Part model, mm, in its own coordinate system. Face numbers are marked on the shaded views. A direction names the side the tool comes from. Round coordinates to 2 decimals unless told otherwise and drop trailing zeros. Loops run counter-clockwise (first coordinate to the right, second up) from the corner with the lowest first, then second, coordinate; pieces in that order, holes last.
(1) Probe probe 1 along Z at (x, y) = (-0.9, 1.25); probe 2 along Z at (x, y) = (-0.65, -0.5) (3 decimals); probe 3 along Y at (x, z) = (0.4, 1.75). List the from-to ranges inside material, lowest first.
(2) Tool access for the marked faces 1 and 2: list every direction of +Z, -Z, +X, -X, +Y, -Y with a clear straight run to the whole face (end or side of a thin tool).
(3) Cut at A-A on z = -2. List the corners of the cut face in (x, y), then the cut area to 3 significant figures.
(4) Mould opens along X. For the marked faces 3, 4, 5 and 6 say: +X half, -X half, draft (parallel to the pull), parting line (faces both ways), or undercut.
(5) Flat gauge pins, fed straight in: pin 1 (1.2 mm diameter, centred on x = 0, y = 0, fed in from +Z); pin 2 (1.5 mm diameter, centred on x = -1, z = -0.5, fed in from -Y). Where does each tip first touch, or does it go through?
Autodesk Inventor part; units mm, degrees
ref_plane "YZ Plane" through (0, 0, 0) normal (1, 0, 0) x (0, 1, 0)
ref_plane "XZ Plane" through (0, 0, 0) normal (0, 1, 0) x (-1, 0, 0)
ref_plane "XY Plane" through (0, 0, 0) normal (0, 0, 1) x (1, 0, 0)
sketch "Sketch1" plane through (0, 0, 0) normal (0, 0, 1) x (1, 0, 0)
  circle A0 centre (0, 0) radius 2.3241
  dimension "max_head_dia" = 4.6482
extrude "Extrusion1" add sketch "Sketch1" along normal blind 2.8448
sketch "Sketch2" plane through (0, 0, 0) normal (0, 0, -1) x (-1, 0, 0)
  circle A0 centre (0, 0) radius 2.3241
  circle A1 centre (0, 0) radius 1.4224
  dimension "max_body_dia" = 2.8448
extrude "Extrusion2" add sketch "Sketch2" along normal blind 9.525 contours A1
sketch "Sketch3" plane through (0, 0, 2.8448) normal (0, 0, 1) x (1, 0, 0)
  circle A0 centre (0, 0) radius 2.3241
  line L0 (-1.1397, 0.7689) -> (0.096, 1.3715)
  line L1 (0.096, 1.3715) -> (1.2357, 0.6026)
  line L2 (1.2357, 0.6026) -> (1.1397, -0.7689)
  line L3 (1.1397, -0.7689) -> (-0.096, -1.3715)
  line L4 (-0.096, -1.3715) -> (-1.2357, -0.6026)
  line L5 (-1.2357, -0.6026) -> (-1.1397, 0.7689)
  dimension "hex_socket_size" = 2.3813
extrude "Extrusion3" cut sketch "Sketch3" against normal blind 1.2954 contours L0 L1 L2 L3 L4 L5
thread "Thread1"
chamfer "Chamfer1" distance 0.254 angle 45 1 edges at (1.4224, 0, -9.525)
fillet "Fillet1" radius 0.127 1 edges at (-2.3241, 0, 2.8448)
fillet "Fillet2" radius 0.127 1 edges at (-2.3241, 0, 0)
fillet "Fillet3" radius 0.127 6 edges at (-1.1877, 0.0832, 2.8448) (-0.5218, 1.0702, 2.8448) (0.6659, 0.987, 2.8448) (1.1877, -0.0832, 2.8448) (0.5218, -1.0702, 2.8448) (-0.6659, -0.987, 2.8448)
properties part number "4_40_hex_cap_screw"
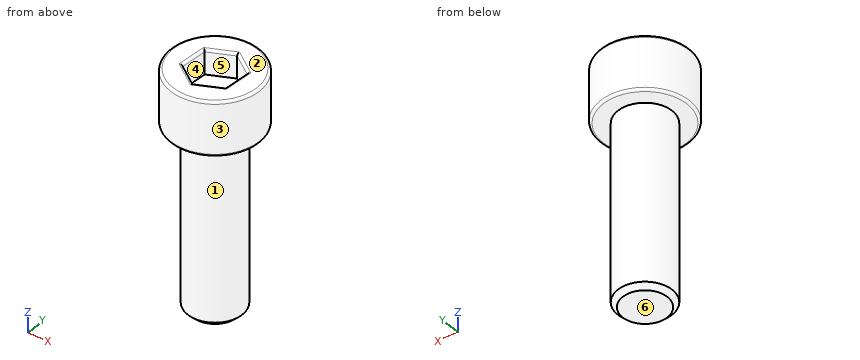
Final values:
1. probe 1: z = 0 to 2.84
1. probe 2: z = -9.525 to 1.549
1. probe 3: y = -2.29 to -1.13, 1.17 to 2.29
2. face 1: -Z
2. face 2: +Z, +X, -X, +Y, -Y
3. outline: circle Ø2.84 at (0, 0)
3. area: 6.36 mm2
4. face 3: parting line
4. face 4: undercut
4. face 5: undercut
4. face 6: draft
5. pin 1: stops at z = 1.55
5. pin 2: stops at y = -2.26
